Part model, mm, in its own coordinate system. A direction names the side the tool comes from. Give positions to 0.01 mm unless a question says otherwise; leave off trailing zeros. Order: outer loops, then holes, each group sorted by start corner. A loop starts at its lowest first (then second) coordinate and runs counter-clockwise, first axis right, second up. Notation, with made-up numbers: (50, 32) - (92, 32) arc R25 ccw to (92, 46) - close; hole circle Ø9 at (89.5, 32.5). An arc over 180 degrees is marked (long way). Use a Markdown table: item, result. Add a question column.
from build123d import *

# Parameters (mm, degrees)
SKETCH1_W                                      = 50
SKETCH1_H                                      = 50
BOSS_EXTRUDE1_DEPTH                            = 40
SHELL1_T                                       = -2.5
SKETCH2_W                                      = 14
SKETCH2_H                                      = 45
BOSS_EXTRUDE2_DEPTH                            = 7
SKETCH4_W                                      = 10.8
SKETCH4_H                                      = 30.2
CUT_EXTRUDE1_DEPTH                             = 6.2
CSK_SLOT_FOR_M1_6_COUNTERSUNK_FLAT_H_2_COUNT   = 2
CSK_SLOT_FOR_M1_6_COUNTERSUNK_FLAT_H_2_PITCH   = 22
CUT_EXTRUDE4_REACH                             = 48.693
SKETCH11_W                                     = 14
SKETCH11_H                                     = 12
SKETCH19_W                                     = 14
SKETCH19_H                                     = 30.5
BOSS_EXTRUDE5_DEPTH                            = 6.5
SKETCH20_W                                     = 10.8
SKETCH20_H                                     = 30.2
CUT_EXTRUDE6_DEPTH                             = 6.2
CSK_SLOT_FOR_M1_6_COUNTERSUNK_FLAT_H_3_A_COUNT = 2
CSK_SLOT_FOR_M1_6_COUNTERSUNK_FLAT_H_3_A_PITCH = 22
SKETCH30_W                                     = 4
SKETCH30_H                                     = 4
BOSS_EXTRUDE6_DEPTH                            = 37.5
CUT_EXTRUDE8_REACH                             = 66.37
SKETCH33_R                                     = 3
SKETCH35_W                                     = 14
SKETCH35_H                                     = 10
CUT_EXTRUDE10_DEPTH                            = 10


with BuildPart() as part:
    # Sketch1 → Boss-Extrude1 (new body)
    with BuildSketch(Plane(origin=(0, 0, 0), x_dir=(1, 0, 0), z_dir=(0, 1, 0))):
        Rectangle(SKETCH1_W, SKETCH1_H)
    extrude(amount=BOSS_EXTRUDE1_DEPTH)

    # Shell1
    shell1_openings = [part.faces().sort_by_distance(p)[0] for p in [
        (0, 40, 0),
    ]]
    offset(amount=SHELL1_T, openings=shell1_openings, kind=Kind.INTERSECTION)

    # Sketch2 → Boss-Extrude2 (add)
    with BuildSketch(Plane(origin=(0, 2.5, 0), x_dir=(1, 0, 0), z_dir=(0, 1, 0))):
        Rectangle(SKETCH2_W, SKETCH2_H)
    extrude(amount=BOSS_EXTRUDE2_DEPTH)

    # Sketch4 → Cut-Extrude1 (cut)
    with BuildSketch(Plane.XZ):
        Rectangle(SKETCH4_W, SKETCH4_H)
    extrude(amount=-CUT_EXTRUDE1_DEPTH, mode=Mode.SUBTRACT)

    # Sketch7 → CSK SLOT for M1.6 Countersunk Flat Head (revolve, cut)
    with BuildSketch(Plane(origin=(0, 9.5, -11), x_dir=(0, 0, 1), z_dir=(1, 0, 0))):
        Polygon((0, 0), (0, 9.5), (0.9, 9.5), (0.9, 2.9), (1.8, 2), (1.8, 0), align=None)
    csk_slot_for_m1_6_countersunk_flat_head = revolve(axis=Axis((0, 15.85, -11), (0, -1, 0)), mode=Mode.SUBTRACT)

    # CSK SLOT for M1.6 Countersunk Flat H 2: CSK SLOT for M1.6 Countersunk Flat Head ×2
    with Locations(*[(0, 0, i * CSK_SLOT_FOR_M1_6_COUNTERSUNK_FLAT_H_2_PITCH) for i in range(1, CSK_SLOT_FOR_M1_6_COUNTERSUNK_FLAT_H_2_COUNT)]):
        add(csk_slot_for_m1_6_countersunk_flat_head, mode=Mode.SUBTRACT)

    # Cut-Extrude4: up to this face of the body (flat: up to its plane)
    cut_extrude4_end = Plane(part.part.faces().sort_by_distance((-14.75, 2.5, 0))[0])
    # Sketch11 → Cut-Extrude4 (cut, up to the picked face)
    with BuildSketch(Plane(origin=(0, 9.5, 0), x_dir=(1, 0, 0), z_dir=(0, 1, 0)), mode=Mode.PRIVATE) as cut_extrude4_sk1:
        Rectangle(SKETCH11_W, SKETCH11_H)
    cut_extrude4_tool1 = split(extrude(cut_extrude4_sk1.sketch, amount=-CUT_EXTRUDE4_REACH, mode=Mode.PRIVATE), bisect_by=cut_extrude4_end, keep=Keep.BOTH, mode=Mode.PRIVATE)
    add(cut_extrude4_tool1.solids().sort_by(Axis((0, 9.5, 0), (0, -1, 0)))[0], mode=Mode.SUBTRACT)

    # Sketch19 → Boss-Extrude5 (add)
    with BuildSketch(Plane.XY.offset(-22.5)):
        with Locations((0, 24.75)):
            Rectangle(SKETCH19_W, SKETCH19_H)
    extrude(amount=BOSS_EXTRUDE5_DEPTH)

    # Sketch20 → Cut-Extrude6 (cut)
    with BuildSketch(Plane(origin=(0, 0, -25), x_dir=(-1, 0, 0), z_dir=(0, 0, -1))):
        with Locations((0, 25)):
            Rectangle(SKETCH20_W, SKETCH20_H)
    extrude(amount=-CUT_EXTRUDE6_DEPTH, mode=Mode.SUBTRACT)

    # Sketch27 → CSK SLOT for M1.6 Countersunk Flat H 3 (revolve, cut)
    with BuildSketch(Plane(origin=(0, 36, -16), x_dir=(0, -1, 0), z_dir=(1, 0, 0))):
        Polygon((0, 0), (0, 40.540774557), (0.9, 40), (0.9, 2.4), (1.8, 1.5), (1.8, 0), align=None)
    csk_slot_for_m1_6_countersunk_flat_h_3 = revolve(axis=Axis((0, 36, -9.65), (0, 0, -1)), mode=Mode.SUBTRACT)

    # CSK SLOT for M1.6 Countersunk Flat H 3 a: CSK SLOT for M1.6 Countersunk Flat H 3 ×2
    with Locations(*[(0, -i * CSK_SLOT_FOR_M1_6_COUNTERSUNK_FLAT_H_3_A_PITCH, 0) for i in range(1, CSK_SLOT_FOR_M1_6_COUNTERSUNK_FLAT_H_3_A_COUNT)]):
        add(csk_slot_for_m1_6_countersunk_flat_h_3, mode=Mode.SUBTRACT)

    # Sketch30 → Boss-Extrude6 (add)
    with BuildSketch(Plane(origin=(0, 2.5, 0), x_dir=(1, 0, 0), z_dir=(0, 1, 0))):
        with Locations((-20.5, 0)):
            Rectangle(SKETCH30_W, SKETCH30_H)
    boss_extrude6 = extrude(amount=BOSS_EXTRUDE6_DEPTH)

    # Sketch32 → M1.6 Tapped Hole2 (revolve, cut)
    with BuildSketch(Plane(origin=(-20.5, 40, 0), x_dir=(0, 0, 1), z_dir=(1, 0, 0))):
        Polygon((0, 0), (0, 5.375537887), (0.625, 5), (0.625, 0), align=None)
    m1_6_tapped_hole2 = revolve(axis=Axis((-20.5, 46.35, 0), (0, -1, 0)), mode=Mode.SUBTRACT)

    # Mirror3: Boss-Extrude6, M1.6 Tapped Hole2 across plane
    add(boss_extrude6.mirror(Plane(origin=(0, 0, 0), x_dir=(0, 0, 1), z_dir=(1, 0, 0))))
    add(m1_6_tapped_hole2.mirror(Plane(origin=(0, 0, 0), x_dir=(0, 0, 1), z_dir=(1, 0, 0))), mode=Mode.SUBTRACT)

    # Sketch33 → Cut-Extrude8 (cut, up to next)
    with BuildSketch(Plane(origin=(0, 0, -18.8), x_dir=(-1, 0, 0), z_dir=(0, 0, -1)), mode=Mode.PRIVATE) as cut_extrude8_sk1:
        with Locations((0, 25)):
            Circle(SKETCH33_R)
    cut_extrude8_tool1 = extrude(cut_extrude8_sk1.sketch, amount=-CUT_EXTRUDE8_REACH, mode=Mode.PRIVATE) & part.part
    add(cut_extrude8_tool1.solids().sort_by_distance((0, 25, -18.8))[0], mode=Mode.SUBTRACT)

    # Sketch35 → Cut-Extrude10 (cut)
    with BuildSketch(Plane(origin=(0, 0, 22.5), x_dir=(-1, 0, 0), z_dir=(0, 0, -1))):
        with Locations((0, 14.5)):
            Rectangle(SKETCH35_W, SKETCH35_H)
    extrude(amount=-CUT_EXTRUDE10_DEPTH, mode=Mode.SUBTRACT)


solid = part.part
1. Mould opens along X. For faces 5 (the face through (0, 20, 25)), 6 (the face through (21, 21, 2)), 7 (the face through (-25, 20, 0)) say: released by +X, released by -X, zero draft, split by the parting line, or undercut.
2. Cut at B-B (x = 4). Write the cut outline in (y, z), plus the area to 3 significant figures.
3. Cut at C-C (z = 11). Write the cut outline in (x, y), plus the area to 3 significant figures.
4. Cut at D-D (y = 31). Write the cut outline in (x, z).
5. Drill centre lines: probe 1 along X at (y, z) = (17.5, -17); probe 2 along Z at (x, y) = (-19.5, 26); probe 3 along X at (y, z) = (14, -18.45). Where is each one in solid material? Low to high. Write a range as [from, to].
6. Tool access for faces 1 (the face through (0, 3, 15.1)), 2 (the face through (0, 8, -6)), 3 (the face through (-5.4, 25, -22)), 4 (the face through (0.65, 22.07, -17.42)): list every direction of +Z, -Z, +X, -X, +Y, -Y with a clear straight run to the whole face (end or side of a thin tool).
7. Cut at A-A (y = 8.5). Write the cut outline in (x, z).
8. Pin check, flat tips, straight feed: P1, Ø15.5, axis at x = 0.5, z = 12, coming from the +Y side; P2, Ø2.5, axis at x = 0, y = 14, coming from the -Z side; P3, Ø5, axis at x = 19.5, z = -9.5, coming from the +Y side. Stop position of each tip, or through.
Responses:
| question | item | result |
|---|---|---|
| 1 | face 5 | zero draft |
| 1 | face 6 | undercut |
| 1 | face 7 | released by -X |
| 2 | outline | (0, -25) - (9.9, -25) - (9.9, -18.8) - (40, -18.8) - (40, -16) - (9.5, -16) - (9.5, -6) - (6.2, -6) - (6.2, -15.1) - (0, -15.1) - close; (0, 15.1) - (6.2, 15.1) - (6.2, 6) - (9.5, 6) - (9.5, 25) - (0, 25) - close; (19.5, 22.5) - (40, 22.5) - (40, 25) - (19.5, 25) - close |
| 2 | area | 387 mm² |
| 3 | outline | (-25, 0) - (-5.4, 0) - (-5.4, 6.2) - (-0.9, 6.2) - (-0.9, 6.6) - (-1.8, 7.5) - (-1.8, 9.5) - (-7, 9.5) - (-7, 2.5) - (-22.5, 2.5) - (-22.5, 40) - (-25, 40) - close; (0.9, 6.2) - (5.4, 6.2) - (5.4, 0) - (25, 0) - (25, 40) - (22.5, 40) - (22.5, 2.5) - (7, 2.5) - (7, 9.5) - (1.8, 9.5) - (1.8, 7.5) - (0.9, 6.6) - close |
| 3 | area | 333 mm² |
| 4 | outline | (-25, -25) - (-5.4, -25) - (-5.4, -18.8) - (5.4, -18.8) - (5.4, -25) - (25, -25) - (25, 25) - (-25, 25) - close; hole (-22.5, -22.5) - (-7, -22.5) - (-7, -16) - (7, -16) - (7, -22.5) - (22.5, -22.5) - (22.5, -2) - (18.5, -2) - (18.5, 2) - (22.5, 2) - (22.5, 22.5) - (-22.5, 22.5) - (-22.5, 2) - (-18.5, 2) - (-18.5, -2) - (-22.5, -2) - close |
| 5 | probe 1 | x = [-25, -22.5], [-7, 7], [22.5, 25] |
| 5 | probe 2 | z = [-25, -22.5], [-2, 2], [22.5, 25] |
| 5 | probe 3 | x = [-25, -22.5], [-7, -0.9], [0.9, 7], [22.5, 25] |
| 6 | face 1 | -Y |
| 6 | face 2 | +Y |
| 6 | face 3 | -Z, +Y |
| 6 | face 4 | -Z |
| 7 | outline | (-25, -25) - (25, -25) - (25, 25) - (-25, 25) - close; hole (-22.5, -22.5) - (-7, -22.5) - (-7, -6) - (7, -6) - (7, -22.5) - (22.5, -22.5) - (22.5, -2) - (18.5, -2) - (18.5, 2) - (22.5, 2) - (22.5, 22.5) - (7, 22.5) - (7, 6) - (-7, 6) - (-7, 22.5) - (-22.5, 22.5) - (-22.5, 2) - (-18.5, 2) - (-18.5, -2) - (-22.5, -2) - close; hole circle Ø3.6 at (0, -11); hole circle Ø3.6 at (0, 11) |
| 8 | P1 | stops at y = 9.5 |
| 8 | P2 | stops at z = -18.8 |
| 8 | P3 | stops at y = 2.5 |
